from build123d import *

# Parameters (mm, degrees)
SKETCH2_R               = 17.5
SKETCH2_R_2             = 15.9125
BOSS_EXTRUDE1_DEPTH     = 600
SKETCH5_W               = 2.75
SKETCH5_H               = 17.5
MIRROR2_COPY_1_SKETCH_W = 2.75
MIRROR2_COPY_1_SKETCH_H = 17.5
SKETCH6_R               = 2.75
CUT_EXTRUDE1_DEPTH      = 18.5000001
CUT_EXTRUDE1_DEPTH_BACK = 18.5000001


with BuildPart() as part:
    # Sketch2 → Boss-Extrude1 (new body, symmetric)
    with BuildSketch(Plane.XY):
        Circle(SKETCH2_R)
        Circle(SKETCH2_R_2, mode=Mode.SUBTRACT)
    extrude(amount=BOSS_EXTRUDE1_DEPTH, both=True)

    # Sketch5 → M5 Clearance Hole1 (revolve, cut)
    with BuildSketch(Plane(origin=(0, 0, -585), x_dir=(0, 0, -1), z_dir=(1, 0, 0))):
        with Locations((1.375, 8.75)):
            Rectangle(SKETCH5_W, SKETCH5_H)
    m5_clearance_hole1 = revolve(axis=Axis((0, -6.35, -585), (0, 1, 0)), mode=Mode.SUBTRACT)

    # Mirror1: M5 Clearance Hole1 across plane
    add(m5_clearance_hole1.mirror(Plane.ZX), mode=Mode.SUBTRACT)

    # Mirror2: M5 Clearance Hole1 across plane
    add(m5_clearance_hole1.mirror(Plane.XY), mode=Mode.SUBTRACT)

    # Mirror2 copy 1 sketch → Mirror2 copy 1 (revolve, cut)
    with BuildSketch(Plane(origin=(0, 0, 585), x_dir=(0, 0, 1), z_dir=(1, 0, 0))):
        with Locations((1.375, 8.75)):
            Rectangle(MIRROR2_COPY_1_SKETCH_W, MIRROR2_COPY_1_SKETCH_H)
    revolve(axis=Axis((0, 6.35, 585), (0, -1, 0)), mode=Mode.SUBTRACT)

    # Sketch6 → Cut-Extrude1 (cut, two sides)
    with BuildSketch(Plane(origin=(0, 0, 0), x_dir=(1, 0, 0), z_dir=(0, 1, 0))) as cut_extrude1_sk:
        with Locations((0, -361.65)):
            Circle(SKETCH6_R)
    extrude(amount=CUT_EXTRUDE1_DEPTH, mode=Mode.SUBTRACT)
    extrude(cut_extrude1_sk.sketch, amount=-CUT_EXTRUDE1_DEPTH_BACK, mode=Mode.SUBTRACT)


solid = part.part
Could you check a few things on this model? Use its own coordinates, in mm. Coordinates: 2 decimals unless noted, no trailing zeros. Write each loop counter-clockwise with the first axis right and the second up, starting at its lowest first coordinate (ties: lowest second). Pieces come first, ordered by that corner, then holes. Notation, with made-up numbers: (-11, 81) - (4, 81) arc R25 ccw to (4, 100) - close; hole circle Ø2 at (-23.75, -18.5). An arc over 180 degrees is marked (long way). Write item = value, one per line.
1) Will these pins go through, and if not, where does the flat tip stop? pin 1 Ø1 at (x, z) = (-3, 261) entering from +Y; pin 2 Ø10 at (x, z) = (5.5, 128.5) entering from -Y; pin 3 Ø3.5 at (x, z) = (0, 361.65) entering from -Y; pin 4 Ø3 at (y, z) = (-12.5, 223.5) entering from -X.
Result set:
pin_1 = 17.32
pin_2 = -17.49
pin_3 = through
pin_4 = -13.61
2) Suppose I cut it at B-B on z = -129.5. Please give me the cut outline in (x, y) (1 decimal).
Result set:
outline = circle Ø35 at (0, 0); hole circle Ø31.8 at (0, 0)
3) Please list where these lines run through material, in increasing order: line 1 (Z direction, x = 0, y = 16.8); line 2 (Y direction, x = -2, z = -385); line 3 (X direction, y = 1.5, z = 453). Write a range as [from, to].
Result set:
line_1 = [-600, -587.75], [-582.25, 358.9], [364.4, 582.25], [587.75, 600]
line_2 = [-17.39, -15.79], [15.79, 17.39]
line_3 = [-17.44, -15.84], [15.84, 17.44]
4) Suppose I cut it at A-A on y = 0. Please give me the cut outline in (x, z).
Result set:
outline = (-17.5, -600) - (-15.91, -600) - (-15.91, 600) - (-17.5, 600) - close; (15.91, -600) - (17.5, -600) - (17.5, 600) - (15.91, 600) - close
5) We'd pull the mould along Y, two halves only. Please class faces 1 (the flat face through (8, -14, 600)), 2 (the cylindrical face through (-2.071, 15.777, -8.4)), 3 (the cylindrical face through (-13.887, -10.648, 8.4)): +Y half, -Y half, draft (parallel to the pull), parting line (faces both ways), or undercut.
Result set:
face_1 = draft
face_2 = undercut
face_3 = parting line
